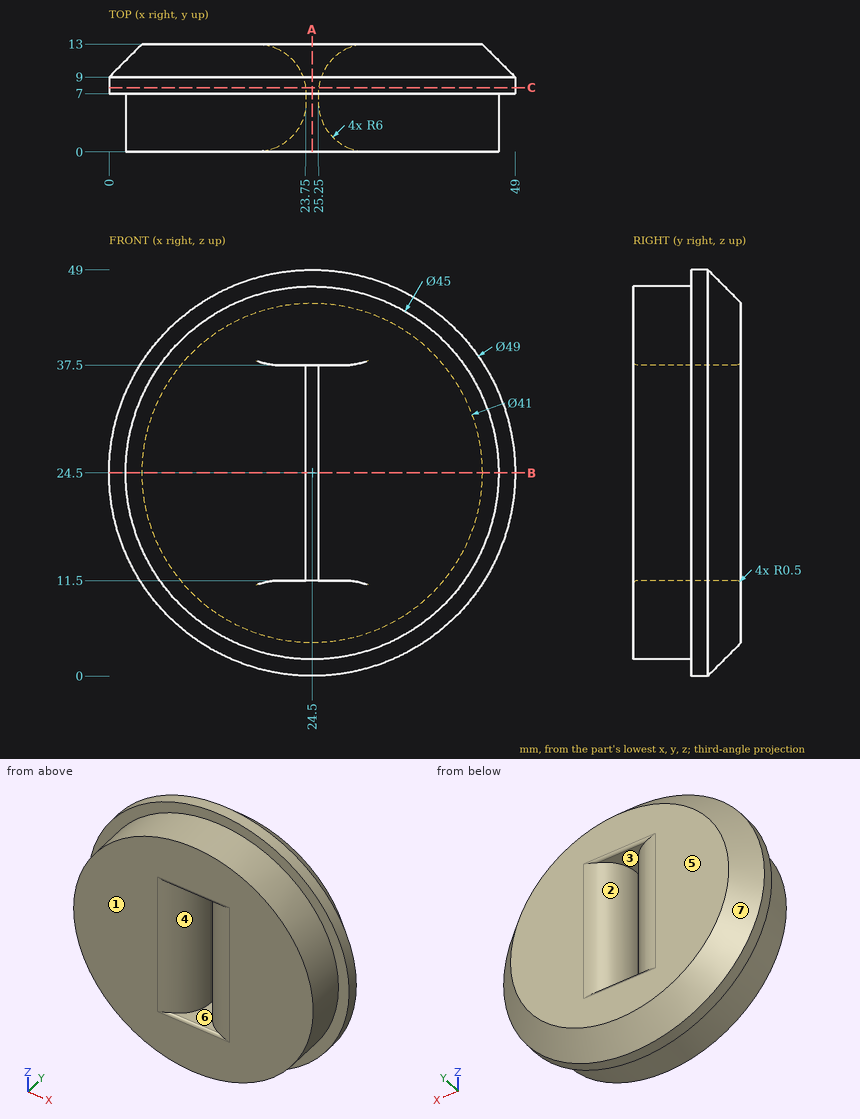
The drawing under review shows one solid part. Ordinate dimensions are in mm from its lowest x, y, z. A direction names the side the tool comes from. Give positions to 0.01 mm unless a question says otherwise; leave off trailing zeros. Write each loop counter-clockwise with the first axis right and the second up, starting at its lowest first coordinate (ties: lowest second). Pieces come first, ordered by that corner, then holes. Notation, with made-up numbers: (20.5, 36) - (65.5, 36) arc R23 cw to (65.5, 50) - close; hole circle Ø7 at (-19.5, 12.5). An arc over 180 degrees is marked (long way). Answer in a Markdown table with one row per item. Add a question column.
1. We need section C-C on y = 7.75. Write out the cut boundary in (x, z).
2. Wall thickness on line 1 along Z through (x, y) = (6.5, 6.5); line 2 along Z through (x, y) = (23, 11); line 3 along X through (y, z) = (5, 18): over which ranges is each line inside the solid? List them lowest first. Write a range as [from, to].
3. Tool access review of the marked faces 1, 2, 3 and 4: name each direction out of +Z, -Z, +X, -X, +Y, -Y from which nothing blocks a thin tool from reaching the whole face with its end or side.
4. Draft analysis for pull direction Z (two halves, no side actions). For the marked faces 5, 6 and 7, state which applies: +Z half, -Z half, draft (parallel to the pull), parting line (faces both ways), or undercut.
5. We need section B-B on z = 24.5. Write out the cut boundary in (x, y), then the cut area to 3 significant figures.
6. We need section A-A on x = 24.5. Write out the cut boundary in (y, z).
7. Insertion check: P1, Ø3, axis at y = 8.5, z = 9.5, coming from the +X side; P2, Ø1.1, axis at y = 6.5, z = 19, coming from the -X side; P3, Ø7, axis at x = 26.5, y = 7.5, coming from the +Z side; P4, Ø8, axis at x = 21.5, z = 26, coming from the -Y side. Each pin has a flat end and moves straight along its axis. Give the tip position at first contact, or say it passes through.
Ans:
| question | item | result |
|---|---|---|
| 1 | outline | circle Ø49 at (24.5, 24.5); hole (23.7, 11.5) - (25.3, 11.5) - (25.3, 37.5) - (23.7, 37.5) - close |
| 2 | line 1 | z = [11, 38] |
| 2 | line 2 | z = [2.05, 11.5], [37.5, 46.95] |
| 2 | line 3 | x = [2.96, 23.67], [25.33, 46.04] |
| 3 | face 1 | +Z, -Z, +X, -X, -Y |
| 3 | face 2 | +Y |
| 3 | face 3 | none |
| 3 | face 4 | -Y |
| 4 | face 5 | draft |
| 4 | face 6 | undercut |
| 4 | face 7 | parting line |
| 5 | outline | (0, 7) - (2, 7) - (2, 0) - (17.75, 0) arc R6 ccw to (23.75, 6) - (23.75, 7) arc R6 ccw to (17.75, 13) - (4, 13) - (0, 9) - close; (25.25, 6) arc R6 ccw to (31.25, 0) - (47, 0) - (47, 7) - (49, 7) - (49, 9) - (45, 13) - (31.25, 13) arc R6 ccw to (25.25, 7) - close |
| 5 | area | 543 mm^2 |
| 6 | outline | (0, 2) - (7, 2) - (7, 0) - (9, 0) - (13, 4) - (13, 11) arc R0.5 ccw to (12.5, 11.5) - (0.5, 11.5) arc R0.5 ccw to (0, 11) - close; (0, 38) arc R0.5 ccw to (0.5, 37.5) - (12.5, 37.5) arc R0.5 ccw to (13, 38) - (13, 45) - (9, 49) - (7, 49) - (7, 47) - (0, 47) - close |
| 7 | P1 | stops at x = 44.95 |
| 7 | P2 | stops at x = 0.57 |
| 7 | P3 | stops at z = 49 |
| 7 | P4 | stops at y = 0 |
